Work out the finished part from the listing and answer in its coordinate system (mm). Face numbers are marked on the shaded views. A direction names the side the tool comes from. Coordinates: 2 decimals unless noted, no trailing zeros. Loops run counter-clockwise (first coordinate to the right, second up) from the corner with the lowest first, then second, coordinate; pieces in that order, holes last. Notation, with made-up numbers: (11.5, 59.5) -> (65.5, 59.5) arc R35 ccw to (65.5, 94.5) -> close; hole circle Ø7 at (42, -15). An arc over 180 degrees is marked (long way). Use a Markdown table: item, result. Add a question column.
Autodesk Inventor part; units mm, degrees
ref_plane "YZ Plane" through (0, 0, 0) normal (1, 0, 0) x (0, 1, 0)
ref_plane "XZ Plane" through (0, 0, 0) normal (0, 1, 0) x (-1, 0, 0)
ref_plane "XY Plane" through (0, 0, 0) normal (0, 0, 1) x (1, 0, 0)
sketch "Sketch1" plane through (0, 0, 0) normal (0, 0, 1) x (1, 0, 0)
  line L0 (0, 0) -> (-69.85, 0)
  line L1 (-69.85, 0) -> (-69.85, 33.02)
  line L2 (-69.85, 33.02) -> (0, 33.02)
  line L3 (0, 33.02) -> (0, 0)
  dimension "d0" = 69.85
  dimension "d1" = 33.02
extrude "Extrusion1" add sketch "Sketch1" along normal blind 22.86
shell "Shell1" thickness 2.54 removed faces 1 at (0, 22.0133, 15.24)
sketch "Sketch2" plane through (0, 0, 22.86) normal (0, 0, 1) x (1, 0, 0)
  line L0 (0, 33.02) -> (-69.85, 33.02)
  line L1 (-69.85, 0) -> (0, 0)
  line L2 (-69.85, 33.02) -> (-69.85, 0)
  line L3 (0, 0) -> (0, 33.02)
  line L4 (-45.212, 16.51) -> (-45.212, 24.765)
  line L5 (-45.212, 24.765) -> (-34.925, 24.765)
  line L6 (-34.925, 8.255) -> (-45.212, 8.255)
  line L7 (-45.212, 8.255) -> (-45.212, 16.51)
  line L8 (-24.638, 16.51) -> (-24.638, 8.255)
  line L9 (-24.638, 8.255) -> (-34.925, 8.255)
  line L10 (-24.638, 16.51) -> (-24.638, 24.765)
  line L11 (-24.638, 24.765) -> (-34.925, 24.765)
extrude "Extrusion2" cut sketch "Sketch2" against normal blind 2.54 contours L4 L5 L11 L10 L8 L9 L6 L7
properties part number "Scanner Case v3"
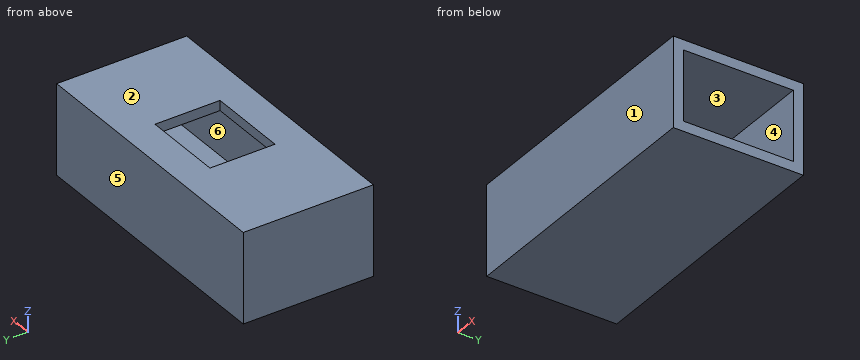
Item 1: Section D-D (y = 28.5) is taken. Determine the outline of the cut face in (x, z), then the cut area to 3 significant figures.
Item 2: For a pull along Z with two mould halves and no side action, classify the marked faces 1, 2, 3 and 4 as +Z half, -Z half, draft (parallel to the pull), parting line (faces both ways), or undercut.
Item 3: Find the intervals of material crossed by probe 1 along Y at (x, z) = (-61, 7.75); probe 2 along X at (y, z) = (11, 3.5); probe 3 along Z at (x, y) = (-14.5, 6.5), in increasing order.
Item 4: Section A-A (y = 19) is taken. Determine the outline of the cut face in (x, z).
Item 5: Section C-C (z = 21.75) is taken. Determine the outline of the cut face in (x, y) (3 decimals), then the cut area to 3 significant figures.
Item 6: For the marked faces 5 and 6, determine the directions among +Z, -Z, +X, -X, +Y, -Y from which every point of the face is accessible in a straight line to the end or side of a thin tool.
Item 7: Section B-B (x = -5) is taken. Determine the outline of the cut face in (y, z), then the cut area to 3 significant figures.
Item 8: Given pin 1 (5.5 mm diameter, centred on y = 17, z = 14.5, fed in from +X), flat-ended and moving along its own axis, determine where the tip first touches the part or whether it passes through.
Output:
| question | item | result |
|---|---|---|
| 1 | outline | (-69.85, 0) -> (0, 0) -> (0, 2.54) -> (-67.31, 2.54) -> (-67.31, 20.32) -> (0, 20.32) -> (0, 22.86) -> (-69.85, 22.86) -> close |
| 1 | area | 400 mm2 |
| 2 | face 1 | draft |
| 2 | face 2 | +Z half |
| 2 | face 3 | undercut |
| 2 | face 4 | undercut |
| 3 | probe 1 | y = 0 to 2.54, 30.48 to 33.02 |
| 3 | probe 2 | x = -69.85 to -67.31 |
| 3 | probe 3 | z = 0 to 2.54, 20.32 to 22.86 |
| 4 | outline | (-69.85, 0) -> (0, 0) -> (0, 2.54) -> (-67.31, 2.54) -> (-67.31, 20.32) -> (-45.21, 20.32) -> (-45.21, 22.86) -> (-69.85, 22.86) -> close; (-24.64, 20.32) -> (0, 20.32) -> (0, 22.86) -> (-24.64, 22.86) -> close |
| 5 | outline | (-69.85, 0) -> (0, 0) -> (0, 33.02) -> (-69.85, 33.02) -> close; hole (-45.212, 8.255) -> (-24.638, 8.255) -> (-24.638, 24.765) -> (-45.212, 24.765) -> close |
| 5 | area | 1,970 mm2 |
| 6 | face 5 | +Z, -Z, +X, -X, +Y |
| 6 | face 6 | +X |
| 7 | outline | (0, 0) -> (33.02, 0) -> (33.02, 22.86) -> (0, 22.86) -> close; hole (2.54, 2.54) -> (30.48, 2.54) -> (30.48, 20.32) -> (2.54, 20.32) -> close |
| 7 | area | 258 mm2 |
| 8 | pin 1 | stops at x = -67.31 |
